from build123d import *

# Parameters (mm, degrees)
SKETCH_3_W          = 10
SKETCH_3_H          = 60
EXTRUDE_3_DEPTH     = 10
SKETCH_4_R          = 10
SKETCH_4_R_2        = 2.6
EXTRUDE_4_DEPTH     = 20
SKETCH_6_W          = 6
SKETCH_6_H          = 50
CUT_EXTRUDE_2_DEPTH = 43.426406871
CUT_EXTRUDE_3_DEPTH = 48.16990566
SKETCH_16_W         = 20
SKETCH_16_H         = 10
EXTRUDE_5_DEPTH     = 20
SKETCH_5_R          = 2.6
CUT_EXTRUDE_1_DEPTH = 46.82575695
SKETCH_18_R         = 2.25
CUT_EXTRUDE_4_DEPTH = 10


with BuildPart() as part:
    # 草图3 → 凸台-拉伸3 (new body)
    with BuildSketch(Plane(origin=(0, 0, 0), x_dir=(1, 0, 0), z_dir=(0, 1, 0))):
        Rectangle(SKETCH_3_W, SKETCH_3_H)
    extrude(amount=EXTRUDE_3_DEPTH)

    # 草图4 → 凸台-拉伸4 (add)
    with BuildSketch(Plane(origin=(0, 0, 0), x_dir=(1, 0, 0), z_dir=(0, 1, 0))):
        with Locations(Location((0, -30, 0), (0, 0, 60))):
            Circle(SKETCH_4_R)
        with Locations(Location((0, -30, 0), (0, 0, 180))):
            Circle(SKETCH_4_R_2, mode=Mode.SUBTRACT)
    extrude(amount=EXTRUDE_4_DEPTH)

    # 草图6 → 切除-拉伸2 (cut, through all)
    with BuildSketch(Plane(origin=(0, 10, 0), x_dir=(1, 0, 0), z_dir=(0, 1, 0))):
        with Locations((3, 5)):
            Rectangle(SKETCH_6_W, SKETCH_6_H)
    extrude(amount=-CUT_EXTRUDE_2_DEPTH, mode=Mode.SUBTRACT)

    # 草图7 → 切除-拉伸3 (cut, through all)
    with BuildSketch(Plane.ZY.offset(5)):
        with BuildLine():
            Line((-27, 6.6), (16, 6.6))
            ThreePointArc((16, 6.6), (17.6, 5), (16, 3.4))
            Line((16, 3.4), (-27, 3.4))
            ThreePointArc((-27, 3.4), (-28.6, 5), (-27, 6.6))
        make_face()
    extrude(amount=-CUT_EXTRUDE_3_DEPTH, mode=Mode.SUBTRACT)

    # 草图16 → 凸台-拉伸5 (add)
    with BuildSketch(Plane.XY.offset(20)):
        with Locations((0, 5)):
            Rectangle(SKETCH_16_W, SKETCH_16_H)
    extrude(amount=EXTRUDE_5_DEPTH)

    # 草图5 → 切除-拉伸1 (cut, through all)
    with BuildSketch(Plane.XZ):
        with Locations(Location((0, 30, 0), (0, 0, 270))):
            Circle(SKETCH_5_R)
    extrude(amount=-CUT_EXTRUDE_1_DEPTH, mode=Mode.SUBTRACT)

    # 草图18 → 切除-拉伸4 (cut)
    with BuildSketch(Plane.XY.offset(40)):
        with Locations((0, 5)):
            Circle(SKETCH_18_R)
    extrude(amount=-CUT_EXTRUDE_4_DEPTH, mode=Mode.SUBTRACT)


solid = part.part
Verification items for the finished model (mm, model axes). A direction names the side the tool comes from. Round coordinates to 2 decimals unless told otherwise and drop trailing zeros. Loops run counter-clockwise (first coordinate to the right, second up) from the corner with the lowest first, then second, coordinate; pieces in that order, holes last. Notation, with made-up numbers: (75, -29) - (130, -29) arc R24 cw to (130, -9) - close; hole circle Ø2 at (58, 60). An arc over 180 degrees is marked (long way). Use a Markdown table: item, result. Add a question column.
1. Section check B-B, the plane y = 5. Record the boundary of the cut face in (x, z), plus the area to 3 significant figures.
2. Access from +Z, -Z, +X, -X, +Y, -Y to the whole of each face (thin tool, end or side, straight path). Record for faces 4 (the face through (-3, 6.6, -6)), 5 (the face through (0, 7, -5)), 6 (the face through (2.146, 5.676, 35.712)).
3. Section check A-A, the plane z = 9.5. Record the boundary of the cut face in (x, y), plus the area to 3 significant figures.
4. Section check D-D, the plane x = 8. Record the boundary of the cut face in (y, z), plus the area to 3 significant figures.
5. Release check for a two-part mould opening along Z. For faces 1 (the face through (8, 10, 38)), 2 (the face through (-2.4, 5.1, 40)), 3 (the face through (0.78, 9.86, 27.52)) record: released by +Z, released by -Z, zero draft, split by the parting line, or undercut.
6. Gauge pin test, flat ends, axial feed: pin 1 (3 mm diameter, centred on y = 7, z = -16, fed in from -X); pin 2 (3 mm diameter, centred on y = 7.5, z = -16.5, fed in from +X); pin 3 (2.5 mm diameter, centred on x = -7.5, y = 2.5, fed in from -Z). Record the tip position at first contact, or that the pin passes through.
7. Section check C-C, the plane x = 1.5. Record the boundary of the cut face in (y, z), plus the area to 3 significant figures.
8. Thickness scan on probe 1 along X at (y, z) = (11, 30); probe 2 along Z at (x, y) = (0, 14.25); probe 3 along Y at (x, z) = (-3.5, -20.5). Record the ranges inside material, lowest first. Write a range as [from, to].
Checks:
| question | item | result |
|---|---|---|
| 1 | outline | (-10, 20) - (-5, 20) - (-5, 17.6) - (0, 17.6) - (0, 20) - (10, 20) - (10, 40) - (2.25, 40) - (2.25, 31.3) arc R2.6 cw (long way) to (-2.25, 31.3) - (-2.25, 40) - (-10, 40) - close; (-5, -30) - (0, -30) - (0, -28.6) - (-5, -28.6) - close |
| 1 | area | 363 mm^2 |
| 2 | face 4 | +X, -X |
| 2 | face 5 | -Z, +X, +Y, -Y |
| 2 | face 6 | +Z |
| 3 | outline | (-5, 0) - (0, 0) - (0, 3.4) - (-5, 3.4) - close; (-5, 6.6) - (0, 6.6) - (0, 10) - (-5, 10) - close |
| 3 | area | 34.0 mm^2 |
| 4 | outline | (0, 20) - (10, 20) - (10, 24) - (20, 24) - (20, 36) - (10, 36) - (10, 40) - (0, 40) - close |
| 4 | area | 320 mm^2 |
| 5 | face 1 | zero draft |
| 5 | face 2 | released by +Z |
| 5 | face 3 | undercut |
| 6 | pin 1 | stops at x = -5 |
| 6 | pin 2 | stops at x = 0 |
| 6 | pin 3 | stops at z = 20 |
| 7 | outline | (0, 20) - (10, 20) - (10, 20.11) - (20, 20.11) - (20, 27.88) - (0, 27.88) - close; (0, 32.12) - (3.32, 32.12) - (3.32, 40) - (0, 40) - close; (6.68, 32.12) - (20, 32.12) - (20, 39.89) - (10, 39.89) - (10, 40) - (6.68, 40) - close |
| 7 | area | 286 mm^2 |
| 8 | probe 1 | x = [-10, -2.6], [2.6, 10] |
| 8 | probe 2 | z = [20, 27.4], [32.6, 40] |
| 8 | probe 3 | y = [0, 3.4], [6.6, 10] |
